Verification items for this drawing (mm, ordinates from the low corner). A direction names the side the tool comes from. Round coordinates to 2 decimals unless told otherwise and drop trailing zeros. Loops run counter-clockwise (first coordinate to the right, second up) from the corner with the lowest first, then second, coordinate; pieces in that order, holes last. Notation, with made-up numbers: (55.25, -39.75) -> (66.25, -39.75) arc R21 cw to (66.25, -1.75) -> close; hole circle Ø4 at (-33, 72). An arc over 180 degrees is marked (long way). Use a Markdown table: item, result. Add a question column.
Q1. Sectioned sample at D-D, the plane x = 3.75. Enter the section's corners in (y, z), then the cut area to 3 significant figures.
Q2. Gauge pin test, flat ends, axial feed: P1, Ø4, axis at x = 7.5, y = 13, coming from the +Z side; P2, Ø1.7, axis at x = 10, y = 10, coming from the -Z side; P3, Ø1, axis at y = 2.5, z = 2.5, coming from the -X side. Record the tip position at first contact, or that the pin passes through.
Q3. Sectioned sample at C-C, the plane z = 7.25. Enter the section's corners in (x, y).
Q4. Sectioned sample at A-A, the plane y = 10. Enter the section's corners in (x, z).
Q5. Material ranges on L1, parallel to Y at x = 10, z = 4.35; L2, parallel to Y at x = 10, z = 6.45; L3, parallel to Z at x = 8.5, y = 12, recorded low to high.
Q6. Release check for a two-part mould opening along X. For the marked faces 1, 2 and 3 record: released by +X, released by -X, zero draft, split by the parting line, or undercut.
Q7. Set-up check for the marked faces 4, 5 and 6: record each of +Z, -Z, +X, -X, +Y, -Y from which the full face is reachable in a straight line by a thin tool's end or side.
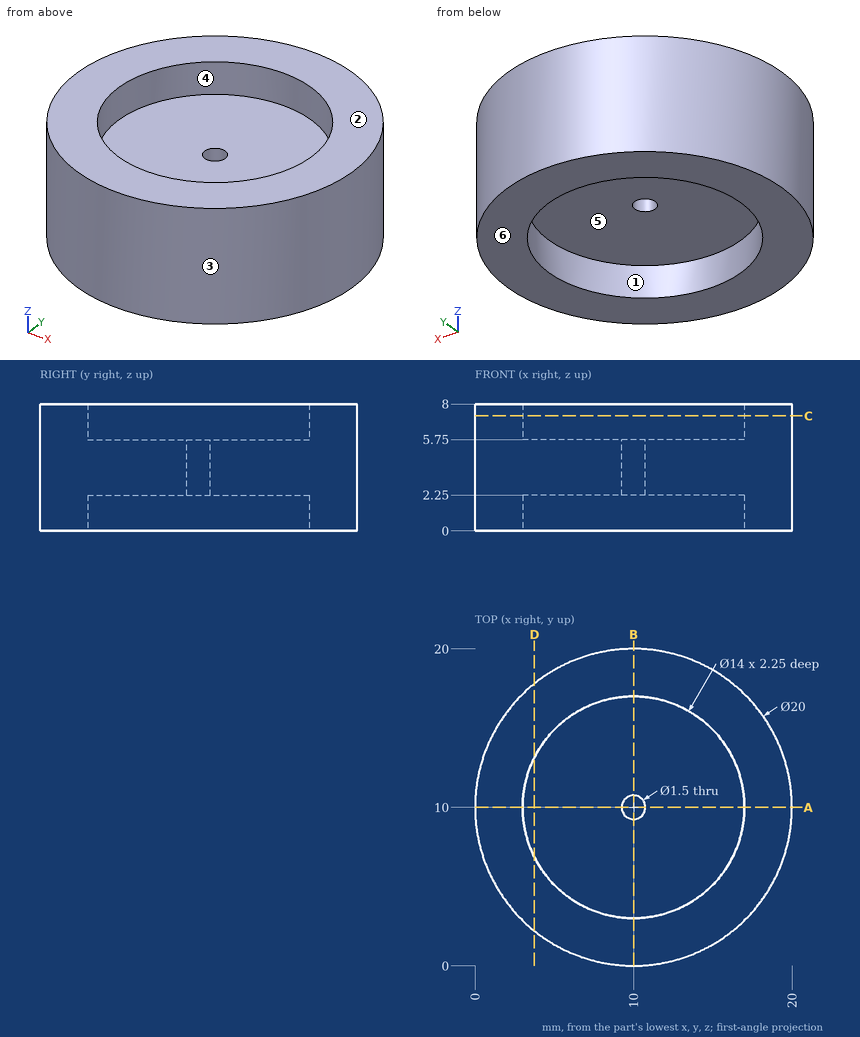
Values:
| question | item | result |
|---|---|---|
| 1 | outline | (2.19, 0) -> (6.85, 0) -> (6.85, 2.25) -> (13.15, 2.25) -> (13.15, 0) -> (17.81, 0) -> (17.81, 8) -> (13.15, 8) -> (13.15, 5.75) -> (6.85, 5.75) -> (6.85, 8) -> (2.19, 8) -> close |
| 1 | area | 96.5 mm^2 |
| 2 | P1 | z = 5.75 |
| 2 | P2 | z = 2.25 |
| 2 | P3 | x = 2.86 |
| 3 | outline | circle Ø20 at (10, 10); hole circle Ø14 at (10, 10) |
| 4 | outline | (0, 0) -> (3, 0) -> (3, 2.25) -> (9.25, 2.25) -> (9.25, 5.75) -> (3, 5.75) -> (3, 8) -> (0, 8) -> close; (10.75, 2.25) -> (17, 2.25) -> (17, 0) -> (20, 0) -> (20, 8) -> (17, 8) -> (17, 5.75) -> (10.75, 5.75) -> close |
| 5 | L1 | 0 to 9.25, 10.75 to 20 |
| 5 | L2 | 0 to 3, 17 to 20 |
| 5 | L3 | 2.25 to 5.75 |
| 6 | face 1 | undercut |
| 6 | face 2 | zero draft |
| 6 | face 3 | split by the parting line |
| 7 | face 4 | +Z |
| 7 | face 5 | -Z |
| 7 | face 6 | -Z, +X, -X, +Y, -Y |
